Check sheet for the drawn part. Datum: minimum x, y, z corner. Units: mm. A direction names the side the tool comes from. Round coordinates to 2 decimals unless told otherwise and drop trailing zeros. Loops run counter-clockwise (first coordinate to the right, second up) from the corner with the lowest first, then second, coordinate; pieces in that order, holes last. Notation, with made-up numbers: (41.5, 67) -> (93.5, 67) arc R27 cw to (93.5, 90) -> close; hole circle Ø6 at (36.25, -1.75). An arc over 180 degrees is marked (long way). Use CSV: the item, a comma, the result in double quotes. Start each with the question number.
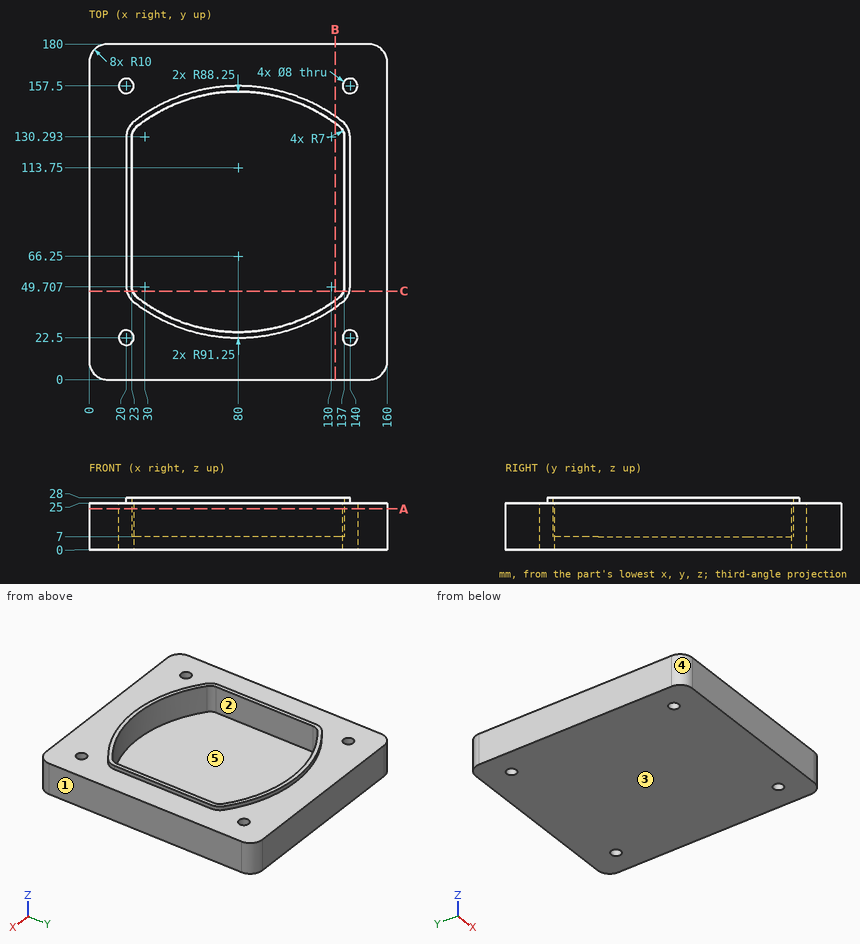
Q1. Depth check by flat-ended pin: pin 1 Ø0.9 at (y, z) = (80, 27) entering from +X. Enter the tip coordinate at first touch or a pass-through.
Q2. Cross-section at B-B (x = 132). Record the boundary of the cut face in (y, z), and give its area (3 significant figures).
Q3. Cross-section at C-C (y = 47.5). Record the boundary of the cut face in (x, z).
Q4. Tool access check on the marked faces 1 and 2. Record the directions out of +Z, -Z, +X, -X, +Y, -Y that give a thin tool (end or side, any length) a straight path to the whole face; none if there is none.
Q5. Thickness scan on L1, parallel to Y at x = 140, z = 11; L2, parallel to X at y = 157.5, z = 16; L3, parallel to X at y = 64, z = 16.5. Record the ranges inside material, lowest first. Write a range as from..to.
Q6. Release check for a two-part mould opening along Y. For the marked faces 3, 4 and 5 record: +Y half, -Y half, draft (parallel to the pull), parting line (faces both ways), or undercut.
Q7. Cross-section at A-A (z = 22). Record the boundary of the cut face in (x, y).
Answer list:
1,pin 1,"stops at x = 140"
2,outline,"(0, 0) -> (180, 0) -> (180, 25) -> (141.23, 25) -> (141.23, 28) -> (137.55, 28) -> (137.55, 7) -> (42.45, 7) -> (42.45, 28) -> (38.77, 28) -> (38.77, 25) -> (0, 25) -> close"
2,area,"2,810 mm2"
3,outline,"(0, 0) -> (160, 0) -> (160, 25) -> (139.75, 25) -> (139.75, 28) -> (136.64, 28) -> (136.64, 7) -> (23.36, 7) -> (23.36, 28) -> (20.25, 28) -> (20.25, 25) -> (0, 25) -> close"
4,face 1,"+Z, -Z, +X, +Y, -Y"
4,face 2,"+Z"
5,L1,"y = 0..18.5, 26.5..153.5, 161.5..180"
5,L2,"x = 0..16, 24..136, 144..160"
5,L3,"x = 0..23, 137..160"
6,face 3,"draft"
6,face 4,"-Y half"
6,face 5,"undercut"
7,outline,"(0, 10) arc R10 ccw to (10, 0) -> (150, 0) arc R10 ccw to (160, 10) -> (160, 170) arc R10 ccw to (150, 180) -> (10, 180) arc R10 ccw to (0, 170) -> close; hole circle Ø8 at (20, 22.5); hole circle Ø8 at (20, 157.5); hole (23, 49.71) arc R7 ccw to (25.69, 44.19) arc R88.25 ccw to (134.31, 44.19) arc R7 ccw to (137, 49.71) -> (137, 130.29) arc R7 ccw to (134.31, 135.81) arc R88.25 ccw to (25.69, 135.81) arc R7 ccw to (23, 130.29) -> close; hole circle Ø8 at (140, 22.5); hole circle Ø8 at (140, 157.5)"
